Build history of the part. All positions in model axes, mm. A direction names the side the tool comes from. Round coordinates to 2 decimals unless told otherwise and drop trailing zeros. Loops run counter-clockwise (first coordinate to the right, second up) from the corner with the lowest first, then second, coordinate; pieces in that order, holes last. Notation, with made-up numbers: (29, 39.25) - (35, 39.25) arc R29 ccw to (35, 67.25) - close; hole circle Ø10 at (85.5, 38.25). An arc over 180 degrees is marked (long way). Put each result on its own line as item: value. Start each with the question number.
Autodesk Inventor part; units mm, degrees
ref_plane "YZ Plane" through (0, 0, 0) normal (1, 0, 0) x (0, 1, 0)
ref_plane "XZ Plane" through (0, 0, 0) normal (0, 1, 0) x (-1, 0, 0)
ref_plane "XY Plane" through (0, 0, 0) normal (0, 0, 1) x (1, 0, 0)
sketch "Skizze1" plane through (0, 0, 0) normal (0, 0, 1) x (1, 0, 0)
  line L0 (-250, 120) -> (250, 120)
  line L1 (250, 120) -> (250, -120)
  line L2 (250, -120) -> (-250, -120)
  line L3 (-250, -120) -> (-250, 120)
  line L4 (-250, 120) -> (250, -120) construction
  line L5 (250, 120) -> (-250, -120) construction
  point P0 (0, 0)
  dimension "d0" = 500
  dimension "d1" = 240
extrude "Extrusion1" add sketch "Skizze1" along normal blind 10
sketch "Skizze2" plane through (0, 0, 10) normal (0, 0, 1) x (1, 0, 0)
  line L0 (-250, 120) -> (-250, -120)
  line L1 (-250, -120) -> (250, -120)
  line L2 (250, -120) -> (250, 120)
  line L3 (-177.5, -100) -> (-155, -15)
  line L4 (-155, -15) -> (-45, -15)
  line L5 (-45, -15) -> (-22.5, -100)
  line L6 (-177.5, -100) -> (-22.5, -100)
  line L7 (143.755, -89) -> (156.245, -89)
  line L8 (169, -76.245) -> (169, -63.755)
  line L9 (156.245, -51) -> (143.755, -51)
  line L10 (131, -63.755) -> (131, -76.245)
  line L11 (143.755, -89) -> (156.245, -51) construction
  line L12 (169, -76.245) -> (131, -63.755) construction
  arc A0 (156.245, -89) -> (169, -76.245) centre (150, -70) ccw
  arc A1 (131, -76.245) -> (143.755, -89) centre (150, -70) ccw
  arc A2 (169, -63.755) -> (156.245, -51) centre (150, -70) ccw
  arc A3 (143.755, -51) -> (131, -63.755) centre (150, -70) ccw
  point P0 (0, 0)
  point P1 (-100, -15)
  point P2 (-100, -100)
  point P3 (-33.75, -57.5)
  dimension "d25" = 155
  dimension "d26" = 110
  dimension "d27" = 150
  dimension "d28" = 20
  dimension "d29" = 85
  dimension "d33" = 100
  dimension "d34" = 50
  dimension "d47" = 38
  dimension "d48" = 20
extrude "Extrusion2" cut sketch "Skizze2" against normal blind 10
sketch "Skizze3" plane through (0, 0, 10) normal (0, 0, 1) x (1, 0, 0)
  circle A0 centre (150, -70) radius 20
  line L0 (134, -86) -> (166, -86)
  line L1 (166, -86) -> (166, -54)
  line L2 (166, -54) -> (134, -54)
  line L3 (134, -54) -> (134, -86)
  line L4 (134, -86) -> (166, -54) construction
  line L5 (166, -86) -> (134, -54) construction
  point P0 (0, 0)
  dimension "d35" = 32
  dimension "d36" = 32
hole "Bohrung3" at (166, -54, 10) at (134, -54, 10) at (134, -86, 10) at (166, -86, 10) direction (0, 0, -1) diameter 2.459 end through all
properties part number "Lid_TopPanel2" material "Polycarbonat, klar"
1) Drop a flat-ended pin along its axis: pin 1 Ø2 at (x, y) = (166, -54) entering from -Z. Give the stop position or say it passes through.
2) Drill centre lines: line 1 (X direction, y = -86, z = 2.75); line 2 (X direction, y = -54, z = 7.75); line 3 (Y direction, x = -82.5, z = 5.5). Where is each one in solid material? Low to high. Write a range as [from, to].
3) Which spindle directions (+Z, -Z, +X, -X, +Y, -Y) get a long thin tool onto all of the face, cutting with end or side? Do faces 5 (the face through (164.234, -55.951, 5.07)), 6 (the face through (3, -120, 5)). Say none if no direction does.
4) Pull direction X, two halves, no side cores. Call faces 1 (the face through (-101, -15, 5)), 2 (the face through (-250, -2, 5)), 3 (the face through (-101, -100, 5)), 4 (the face through (-3, 2, 0)): pulls with the +X half, pulls with the -X half, needs draft (parallel to the pull), parting line crosses it, or undercut.
5) Slice it at A-A, the plane z = 7.5. Write the cut outline in (x, y) (1 decimal).
6) Slice it at B-B, the plane y = -68.5. Write the cut outline in (x, z).
Taken from the geometry:
1. pin 1: passes through
2. line 1: x = [-250, -173.79], [-26.21, 132.77], [135.23, 138], [162, 164.77], [167.23, 250]
2. line 2: x = [-250, -165.32], [-34.68, 132.77], [135.23, 138], [162, 164.77], [167.23, 250]
2. line 3: y = [-120, -100], [-15, 120]
3. face 5: +Z, -Z
3. face 6: +Z, -Z, +X, -X, -Y
4. face 1: undercut
4. face 2: pulls with the -X half
4. face 3: undercut
4. face 4: needs draft
5. outline: (-250, -120) - (250, -120) - (250, 120) - (-250, 120) - close; hole (-177.5, -100) - (-22.5, -100) - (-45, -15) - (-155, -15) - close; hole (131, -76.2) arc R20 ccw to (143.8, -89) - (156.2, -89) arc R20 ccw to (169, -76.2) - (169, -63.8) arc R20 ccw to (156.2, -51) - (143.8, -51) arc R20 ccw to (131, -63.8) - close; hole circle Ø2.5 at (134, -86); hole circle Ø2.5 at (134, -54); hole circle Ø2.5 at (166, -86); hole circle Ø2.5 at (166, -54)
6. outline: (-250, 0) - (-169.16, 0) - (-169.16, 10) - (-250, 10) - close; (-30.84, 0) - (131, 0) - (131, 10) - (-30.84, 10) - close; (169, 0) - (250, 0) - (250, 10) - (169, 10) - close
